from build123d import *

# Parameters (mm, degrees)
BOSS_EXTRUDE1_DEPTH            = 45
SKETCH2_R                      = 12.5
CUT_EXTRUDE1_DEPTH             = 10
SKETCH3_R                      = 12.508139694
CUT_EXTRUDE2_DEPTH             = 15
CUT_EXTRUDE3_REACH             = 53.053
SKETCH4_R                      = 11.5
CUT_EXTRUDE4_REACH             = 53.015
SKETCH5_R                      = 11.5
SM1_TAPPED_HOLE1_D             = 25.4
SM1_TAPPED_HOLE1_DEPTH         = 4
SM1_TAPPED_HOLE1_TIP           = 7.630929862
SM1_TAPPED_HOLE2_D             = 25.4
SM1_TAPPED_HOLE2_DEPTH         = 3.5
SM1_TAPPED_HOLE2_TIP           = 7.630929862
CUT_EXTRUDE5_DEPTH             = 35
SM1_TAPPED_HOLE3_D             = 25.4
SM1_TAPPED_HOLE3_DEPTH         = 5.41
SM1_TAPPED_HOLE3_TIP           = 7.630929862
SM1_TAPPED_HOLE4_D             = 25.4
SM1_TAPPED_HOLE4_DEPTH         = 5.41
SM1_TAPPED_HOLE4_TIP           = 7.630929862
CBORE_FOR_M3_SHCS1_D           = 3.2
CBORE_FOR_M3_SHCS1_DEPTH       = 10
CBORE_FOR_M3_SHCS1_CBORE_D     = 6.5
CBORE_FOR_M3_SHCS1_CBORE_DEPTH = 3
CUT_EXTRUDE6_START             = -5.339235
CUT_EXTRUDE6_DEPTH             = 6
F_3_0MM_DOWEL_HOLE1_D          = 3
F_3_0MM_DOWEL_HOLE1_DEPTH      = 5.2
F_3_0MM_DOWEL_HOLE1_TIP        = 0.901290929
SKETCH21_W                     = 17.451379617
SKETCH21_H                     = 3
SKETCH21_W_2                   = 37.142162435
CUT_EXTRUDE7_DEPTH             = 5.2


with BuildPart() as part:
    # Sketch1 → Boss-Extrude1 (new body)
    with BuildSketch(Plane(origin=(0, 0, 0), x_dir=(1, 0, 0), z_dir=(0, 1, 0))):
        Polygon((5.319745859, 25.342678723), (-23.689372123, 25.342678723), (-23.689372123, 6.626389833), (-46.111095982, -15.795334027), (-60.695537468, -1.210892541), (-38.989042082, 20.495602845), (-38.989042082, 55.962281461), (5.319745859, 55.962281461), align=None)
    extrude(amount=BOSS_EXTRUDE1_DEPTH)

    # Sketch2 → Cut-Extrude1 (cut)
    with BuildSketch(Plane(origin=(-15.157880978, 0, -15.157880978), x_dir=(0.707106781, 0, -0.707106781), z_dir=(0.707106781, 0, 0.707106781))):
        with Locations((-27.941994438, 25.4)):
            Circle(SKETCH2_R)
    extrude(amount=-CUT_EXTRUDE1_DEPTH, mode=Mode.SUBTRACT)

    # Sketch3 → Cut-Extrude2 (cut)
    with BuildSketch(Plane(origin=(5.319745859, 0, 0), x_dir=(0, 0, -1), z_dir=(1, 0, 0))):
        with Locations((40.327918955, 25.4)):
            Circle(SKETCH3_R)
    extrude(amount=-CUT_EXTRUDE2_DEPTH, mode=Mode.SUBTRACT)

    # Sketch4 → Cut-Extrude3 (cut, up to next)
    with BuildSketch(Plane(origin=(-22.228948789, 0, -22.228948789), x_dir=(0.707106781, 0, -0.707106781), z_dir=(0.707106781, 0, 0.707106781)), mode=Mode.PRIVATE) as cut_extrude3_sk1:
        with Locations((-27.941994438, 25.4)):
            Circle(SKETCH4_R)
    cut_extrude3_tool1 = extrude(cut_extrude3_sk1.sketch, amount=-CUT_EXTRUDE3_REACH, mode=Mode.PRIVATE) & part.part
    add(cut_extrude3_tool1.solids().sort_by_distance((-41.986923, 25.4, -2.470975))[0], mode=Mode.SUBTRACT)

    # Sketch5 → Cut-Extrude4 (cut, up to next)
    with BuildSketch(Plane(origin=(-9.680254141, 0, 0), x_dir=(0, 0, -1), z_dir=(1, 0, 0)), mode=Mode.PRIVATE) as cut_extrude4_sk1:
        with Locations((40.327918955, 25.4)):
            Circle(SKETCH5_R)
    cut_extrude4_tool1 = extrude(cut_extrude4_sk1.sketch, amount=-CUT_EXTRUDE4_REACH, mode=Mode.PRIVATE) & part.part
    add(cut_extrude4_tool1.solids().sort_by_distance((-9.680254, 25.4, -40.327919))[0], mode=Mode.SUBTRACT)

    # SM1 Tapped Hole1
    with Locations(Plane(origin=(5.319745859, 0, 0), x_dir=(0, 0, -1), z_dir=(1, 0, 0))):
        with Locations((40.327918955, 25.4)):
            Hole(SM1_TAPPED_HOLE1_D / 2, depth=SM1_TAPPED_HOLE1_DEPTH)
            with Locations((0, 0, -(SM1_TAPPED_HOLE1_DEPTH + SM1_TAPPED_HOLE1_TIP / 2))):  # 118° drill point
                Cone(0, SM1_TAPPED_HOLE1_D / 2, SM1_TAPPED_HOLE1_TIP, mode=Mode.SUBTRACT)

    # SM1 Tapped Hole2
    with Locations(Plane(origin=(-15.157880978, 0, -15.157880978), x_dir=(0.707106781, 0, -0.707106781), z_dir=(0.707106781, 0, 0.707106781))):
        with Locations((-27.941994438, 25.4)):
            Hole(SM1_TAPPED_HOLE2_D / 2, depth=SM1_TAPPED_HOLE2_DEPTH)
            with Locations((0, 0, -(SM1_TAPPED_HOLE2_DEPTH + SM1_TAPPED_HOLE2_TIP / 2))):  # 118° drill point
                Cone(0, SM1_TAPPED_HOLE2_D / 2, SM1_TAPPED_HOLE2_TIP, mode=Mode.SUBTRACT)

    # Sketch11 → Cut-Extrude5 (cut)
    with BuildSketch(Plane(origin=(0, 45, 0), x_dir=(1, 0, 0), z_dir=(0, 1, 0))):
        Polygon((-23.689372123, 6.626389833), (-38.989042082, 20.495602845), (-38.989042082, 55.962281461), (-23.689372123, 55.962281461), align=None)
    extrude(amount=-CUT_EXTRUDE5_DEPTH, mode=Mode.SUBTRACT)

    # SM1 Tapped Hole3
    with Locations(Plane.ZY.offset(23.689372123)):
        with Locations((-40.327918955, 25.4)):
            Hole(SM1_TAPPED_HOLE3_D / 2, depth=SM1_TAPPED_HOLE3_DEPTH)
            with Locations((0, 0, -(SM1_TAPPED_HOLE3_DEPTH + SM1_TAPPED_HOLE3_TIP / 2))):  # 118° drill point
                Cone(0, SM1_TAPPED_HOLE3_D / 2, SM1_TAPPED_HOLE3_TIP, mode=Mode.SUBTRACT)

    # SM1 Tapped Hole4
    with Locations(Plane(origin=(-29.742322464, 0, -29.742322464), x_dir=(-0.707106781, 0, 0.707106781), z_dir=(-0.707106781, 0, -0.707106781))):
        with Locations((27.941994438, 25.4)):
            Hole(SM1_TAPPED_HOLE4_D / 2, depth=SM1_TAPPED_HOLE4_DEPTH)
            with Locations((0, 0, -(SM1_TAPPED_HOLE4_DEPTH + SM1_TAPPED_HOLE4_TIP / 2))):  # 118° drill point
                Cone(0, SM1_TAPPED_HOLE4_D / 2, SM1_TAPPED_HOLE4_TIP, mode=Mode.SUBTRACT)

    # CBORE for M3 SHCS1
    with Locations(Plane(origin=(0, 10, 0), x_dir=(1, 0, 0), z_dir=(0, 1, 0))):
        with Locations((-31.01569247, 48.433741468), (-31.01569247, 21.171407243)):
            CounterBoreHole(CBORE_FOR_M3_SHCS1_D / 2, CBORE_FOR_M3_SHCS1_CBORE_D / 2, CBORE_FOR_M3_SHCS1_CBORE_DEPTH, depth=CBORE_FOR_M3_SHCS1_DEPTH)

    # Sketch18 → Cut-Extrude6 (cut)
    with BuildSketch(Plane.ZY.offset(0.01948891).offset(CUT_EXTRUDE6_START)):
        with BuildLine():
            Line((-46.204849494, 45), (-56.766756342, 45))
            Line((-56.766756342, 45), (-56.766756342, 28.086826547))
            ThreePointArc((-56.766756342, 28.086826547), (-53.24503426, 37.642014764), (-46.204849494, 45))
        make_face()
        with BuildLine():
            Line((-56.619620621, 19.834105942), (-56.619620621, 0))
            Line((-56.619620621, 0), (-37.484367562, 0))
            ThreePointArc((-37.484367562, 0), (-50.031901767, 7.042142066), (-56.619620621, 19.834105942))
        make_face()
    extrude(amount=CUT_EXTRUDE6_DEPTH, mode=Mode.SUBTRACT)

    # Ø3.0mm Dowel Hole1
    with Locations(Plane(origin=(0, 0, 0), x_dir=(-1, 0, 0), z_dir=(0, -1, 0))):
        with Locations((42.575562076, 1.882335503), (30.989042082, 35.462281461)):
            Hole(F_3_0MM_DOWEL_HOLE1_D / 2, depth=F_3_0MM_DOWEL_HOLE1_DEPTH)
            with Locations((0, 0, -(F_3_0MM_DOWEL_HOLE1_DEPTH + F_3_0MM_DOWEL_HOLE1_TIP / 2))):  # 118° drill point
                Cone(0, F_3_0MM_DOWEL_HOLE1_D / 2, F_3_0MM_DOWEL_HOLE1_TIP, mode=Mode.SUBTRACT)

    # Sketch21 → Cut-Extrude7 (cut)
    with BuildSketch(Plane.XZ):
        with Locations((-33.849872268, -1.882335503)):
            Rectangle(SKETCH21_W, SKETCH21_H)
        with Locations((-12.417960864, -35.462281461)):
            Rectangle(SKETCH21_W_2, SKETCH21_H)
    extrude(amount=-CUT_EXTRUDE7_DEPTH, mode=Mode.SUBTRACT)


solid = part.part
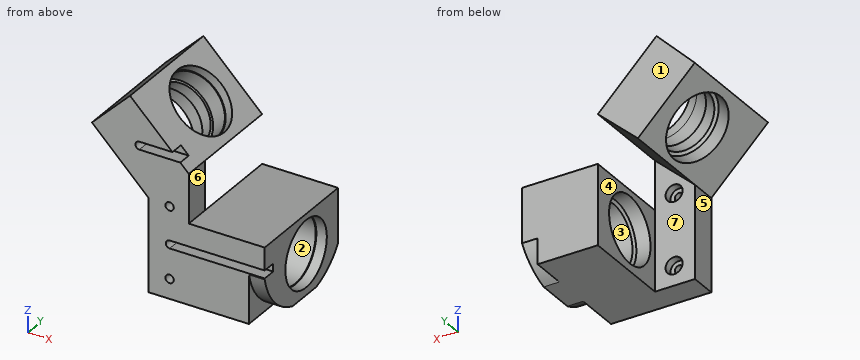
Read the model definition and answer for the solid it produces. Units are mm, in the model's axes. Face numbers are marked on the shaded views. A direction names the side the tool comes from. Coordinates: 2 decimals unless noted, no trailing zeros. Loops run counter-clockwise (first coordinate to the right, second up) from the corner with the lowest first, then second, coordinate; pieces in that order, holes last.
Q1. The mould has two halves that part along Y. Classify the marked faces 1, 2, 3 and 4: +Y half, -Y half, draft (parallel to the pull), parting line (faces both ways), or undercut.
Q2. The part is cut by section C-C on y = 25.4. Give the number of separate pieces and of enclosed holes in the cut face, and give its area (3 significant figures).
Q3. The part is cut by section A-A on x = -14.5. Write down the section's boundary in (y, z).
Q4. Consider probe 1 along Z at (x, y) = (-13.5, 25.4); probe 2 along Z at (x, y) = (3, 25); probe 3 along Z at (x, y) = (-23, 42). Determine where each line is inside the solid, lowest interval first.
Q5. Which of the six approach directions +Z, -Z, +X, -X, +Y, -Y give full straight-line access (tool end or side, diameter ignored) to the marked faces 5, 6 and 7?
Q6. The part is cut by section B-B on y = 8.5. Write down the section's boundary in (x, z), and give its area (3 significant figures).
Q7. Each of these flat-tipped pins is pushed along its axis until it touches: pin 1 Ø1.9 at (x, z) = (-31.02, -21.17) entering from +Y; pin 2 Ø2 at (y, z) = (6.5, -30.5) entering from -X; pin 3 Ø1 at (x, y) = (-10.5, 30.5) entering from +Z; pin 4 Ø11 at (y, z) = (4.5, -12) entering from +X. Where does it stop, or does it pass through?
Results below:
1. face 1: +Y half
1. face 2: undercut
1. face 3: undercut
1. face 4: draft
2. separate pieces: 4
2. enclosed holes: 0
2. area: 309 mm2
3. outline: (0, -55.96) - (45, -55.96) - (45, -25.34) - (0, -25.34) - (0, -33.96) - (5.2, -33.96) - (5.2, -36.96) - (0, -36.96) - close; hole circle Ø23 at (25.4, -40.33)
4. probe 1: z = -55.96 to -51.83, -28.83 to -25.34
4. probe 2: z = -55.96 to -53.02, -27.63 to -25.34
4. probe 3: z = -55.96 to -25.34
5. face 5: -Z, -X, +Y, -Y
5. face 6: +Z, +X, +Y, -Y
5. face 7: -Z, +Y
6. outline: (-60.7, 1.21) - (-38.99, -20.5) - (-38.99, -55.96) - (-0.68, -55.96) - (-0.68, -51.33) - (5.32, -51.33) - (5.32, -25.34) - (-23.69, -25.34) - (-23.69, -6.63) - (-46.11, 15.8) - close; hole circle Ø6.5 at (-31.02, -48.43); hole circle Ø6.5 at (-31.02, -21.17)
6. area: 2,090 mm2
7. pin 1: passes through
7. pin 2: stops at x = -38.99
7. pin 3: stops at z = -25.34
7. pin 4: stops at x = -23.69
